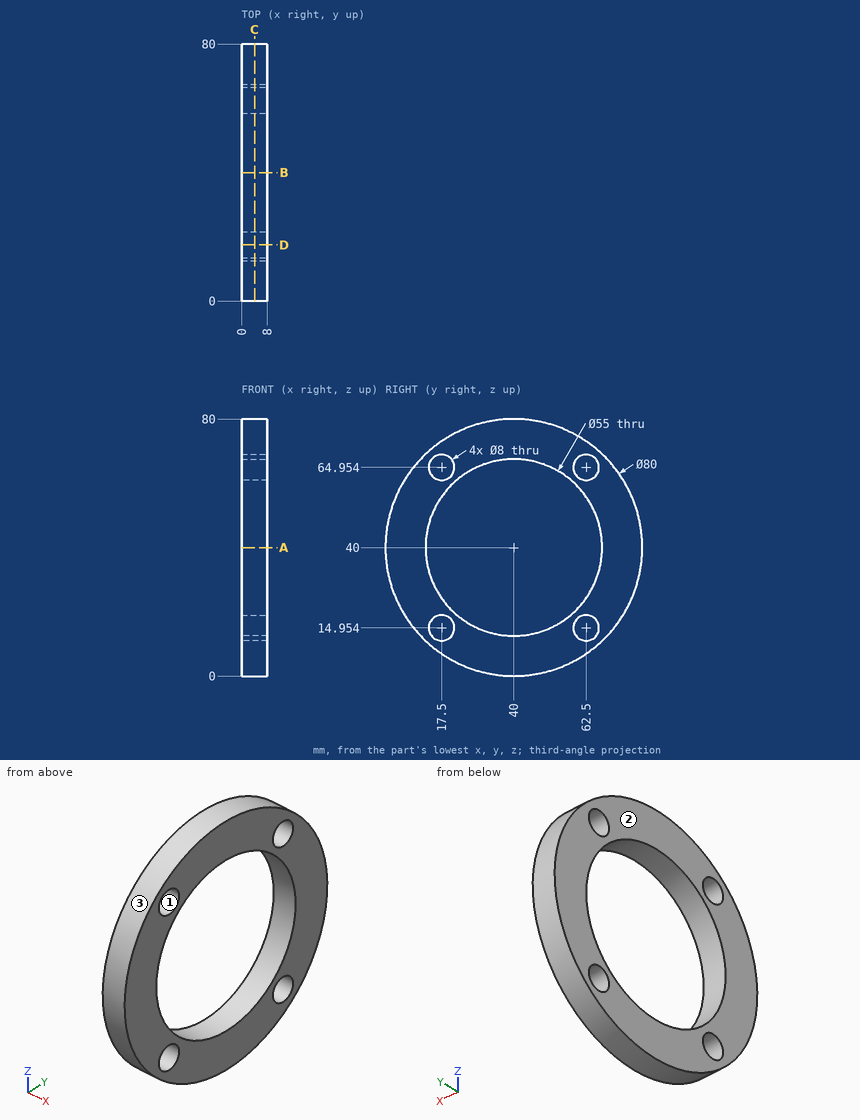
Input: dimensioned drawing with shaded views. Units: mm. Origin: part minimum x, y, z. Coordinates: 2 decimals unless noted, no trailing zeros. Loops run counter-clockwise (first coordinate to the right, second up) from the corner with the lowest first, then second, coordinate; pieces in that order, holes last. Notation, with made-up numbers: M -27,-36 L -5,-36 A27 ccw -5,-7 Z; hole C 36.25,5.5 d8. An arc over 180 degrees is marked long. One line per item, written item: value. Start each with the question number.
1) Cut plane A-A (z = 40). Return loops of the section in (x, y), then the cut area to 3 significant figures.
2) Cut plane D-D (y = 17.5). Return loops of the section in (x, z).
3) Material intervals for L1, parallel to Y at x = 0.5, z = 18; L2, parallel to Z at x = 3.25, y = 39.5; L3, parallel to Z at x = 6.25, y = 65.5 (1 decimal), sorted ascending. Write a range as from..to.
4) Cut plane C-C (x = 4). Return loops of the section in (y, z).
5) Draft query along Z for the marked faces 1, 2 and 3. Return one class per face: released by +Z, released by -Z, zero draft, split by the parting line, or undercut.
6) Pin query (flat end, axial travel): P1, Ø1.5, axis at x = 4, z = 12.5, coming from the +Y side; P2, Ø1, axis at x = 4.5, z = 34, coming from the +Y side. Return the tip coordinate at first contact, or that it passes through.
Evaluation:
1. outline: M 0,0 L 8,0 L 8,12.5 L 0,12.5 Z; M 0,67.5 L 8,67.5 L 8,80 L 0,80 Z
1. area: 200 mm^2
2. outline: M 0,6.93 L 8,6.93 L 8,10.95 L 0,10.95 Z; M 0,18.95 L 8,18.95 L 8,24.19 L 0,24.19 Z; M 0,55.81 L 8,55.81 L 8,60.95 L 0,60.95 Z; M 0,68.95 L 8,68.95 L 8,73.07 L 0,73.07 Z
3. L1: 6.59..14.91, 20.09..23.5, 56.5..59.91, 65.09..73.41
3. L2: 0..12.5, 67.5..80
3. L3: 9.2..12.3, 17.6..29.7, 50.3..62.3, 67.6..70.8
4. outline: C 40,40 d80; hole C 40,40 d55; hole C 17.5,14.95 d8; hole C 17.5,64.95 d8; hole C 62.5,14.95 d8; hole C 62.5,64.95 d8
5. face 1: undercut
5. face 2: zero draft
5. face 3: split by the parting line
6. P1: y = 69.74
6. P2: y = 79.62
